Geometry: final body of the model. Coordinates: model frame, mm. A direction names the side the tool comes from. Coordinates: 2 decimals unless noted, no trailing zeros. Order: outer loops, then holes, each group sorted by start corner. A loop starts at its lowest first (then second) coordinate and runs counter-clockwise, first axis right, second up. Notation, with made-up numbers: (87.5, -4.75) - (141.5, -4.75) arc R20 cw to (141.5, 24.25) - close; hole circle Ø2 at (40.5, -12.75). An arc over 180 degrees is marked (long way). Use a Markdown table: item, result. Add a question column.
```python
from build123d import *

# Parameters (mm, degrees)
CROQUIS1_R              = 10
SALIENTE_EXTRUIR2_DEPTH = 50
CROQUIS4_R              = 30
SALIENTE_EXTRUIR3_DEPTH = 3
SALIENTE_EXTRUIR4_START = 25
CROQUIS5_R              = 30
SALIENTE_EXTRUIR4_DEPTH = 3
REDONDEO2_R             = 10
CORTAR_EXTRUIR1_START   = 50
CORTAR_EXTRUIR1_DEPTH   = 20
CORTAR_EXTRUIR2_START   = 50
CROQUIS7_W              = 3.5
CROQUIS7_H              = 7.2
CORTAR_EXTRUIR2_DEPTH   = 10
CORTAR_EXTRUIR3_START   = 1.785357468
CORTAR_EXTRUIR3_DEPTH   = 8.214642632
CORTAR_EXTRUIR4_START   = 25
CROQUIS9_R              = 2
CORTAR_EXTRUIR4_DEPTH   = 3
REDONDEO3_R             = 3


# Read off the part's stored shape, not the designer's step: Cortar-Extruir3
with BuildPart() as part:
    # Croquis1 → Saliente-Extruir2 (new body)
    with BuildSketch(Plane.XY):
        Circle(CROQUIS1_R)
    extrude(amount=SALIENTE_EXTRUIR2_DEPTH)

    # Croquis4 → Saliente-Extruir3 (add)
    with BuildSketch(Plane.XY):
        Circle(CROQUIS4_R)
    extrude(amount=SALIENTE_EXTRUIR3_DEPTH)

    # Croquis5 → Saliente-Extruir4 (add)
    with BuildSketch(Plane.XY.offset(SALIENTE_EXTRUIR4_START)):
        Circle(CROQUIS5_R)
    extrude(amount=SALIENTE_EXTRUIR4_DEPTH)

    # Redondeo2
    redondeo2_edges = [part.edges().sort_by_distance(p)[0] for p in [
        (-10, 0, 25),
        (-10, 0, 3),
    ]]
    fillet(redondeo2_edges, radius=REDONDEO2_R)

    # Croquis6 → Cortar-Extruir1 (cut)
    with BuildSketch(Plane.XY.offset(CORTAR_EXTRUIR1_START)):
        with BuildLine():
            Line((2, 1.5), (2, -1.5))
            ThreePointArc((2, -1.5), (-2.5, 0), (2, 1.5))
        make_face()
    extrude(amount=-CORTAR_EXTRUIR1_DEPTH, mode=Mode.SUBTRACT)

    # Croquis7 → Cortar-Extruir2 (cut)
    with BuildSketch(Plane.XY.offset(CORTAR_EXTRUIR2_START)):
        with Locations((5.5, 0)):
            Rectangle(CROQUIS7_W, CROQUIS7_H)
    extrude(amount=-CORTAR_EXTRUIR2_DEPTH, mode=Mode.SUBTRACT)

    # Cortar-Extruir3 outline → Cortar-Extruir3 (cut)
    with BuildSketch(Plane(origin=(0, 0, 0), x_dir=(0, 0, -1), z_dir=(1, 0, 0)).offset(CORTAR_EXTRUIR3_START)):
        with BuildLine():
            add(Edge.make_bspline(
                [(-43.250000008, 0), (-43.250010298, 0.457042806), (-43.439269311, 0.91355666), (-44.08377392, 1.559232298), (-44.536167579, 1.749638189), (-45.461098225, 1.750360744), (-45.914256169, 1.560125471), (-46.558728463, 0.916635921), (-46.75, 0.463408547), (-46.75, -0.463408547), (-46.559497121, -0.915462774), (-45.915045576, -1.559741953), (-45.458501244, -1.749734355), (-44.543528816, -1.750265056), (-44.088756623, -1.563446648), (-43.437067231, -0.912124478), (-43.250180582, -0.457964068), (-43.250000045, -0.000460382), (-43.250000003, -0.000230191), (-43.250000008, 0)],
                knots=[0.500062925, 0.500062925, 0.500062925, 0.500062925, 0.625, 0.625, 0.750000001, 0.750000001, 0.875000002, 0.875000002, 1.000000004, 1.000000004, 1.125000006, 1.125000006, 1.250000009, 1.250000009, 1.375000013, 1.375000013, 1.500000015, 1.500000015, 1.50006294, 1.50006294, 1.50006294, 1.50006294], degree=3))
        make_face()
    extrude(amount=CORTAR_EXTRUIR3_DEPTH, mode=Mode.SUBTRACT)

    # Croquis9 → Cortar-Extruir4 (cut)
    with BuildSketch(Plane.XY.offset(CORTAR_EXTRUIR4_START)):
        with Locations((25, 0)):
            Circle(CROQUIS9_R)
    extrude(amount=CORTAR_EXTRUIR4_DEPTH, mode=Mode.SUBTRACT)

    # Redondeo3
    redondeo3_edges = [part.edges().sort_by_distance(p)[0] for p in [
        (-10, 0, 28),
    ]]
    fillet(redondeo3_edges, radius=REDONDEO3_R)


solid = part.part
```
1) Draft query along X for faces 4 (the face through (-2.17, -9.76, 13.99)), 5 (the face through (-2, -2, 50)), 6 (the face through (23, 0, 26)). Return one class per face: pulls with the +X half, pulls with the -X half, needs draft (parallel to the pull), parting line crosses it, or undercut.
2) Set-up query: faces 1 (the face through (-29.97, 1.32, 26.48)), 2 (the face through (5, 3.6, 45)), 3 (the face through (6, -20, 3)). Return all of +Z, -Z, +X, -X, +Y, -Y with unobstructed straight access to the full face (end or side cutting, diameter ignored); none if empty.
3) Section A-A (x = 0). Return loops of the section in (y, z).
4) Section B-B (y = 0). Give the number of separate pieces and of enclosed holes in the cut face, then the cut area to 3 significant figures.
5) Pin query (flat end, axial travel): pin 1 (4 mm diameter, centred on x = 5.5, z = 44.5, fed in from -Y); pin 2 (2 mm diameter, centred on y = -1.5, z = 44, fed in from -X); pin 3 (3 mm diameter, centred on x = 0, y = 0, fed in from +Z). Return the tip coordinate at first contact, or that it passes through.
6) Ray query, line 1 along Z through (x, y) = (-23, -11); line 2 along X through (y, z) = (0, 37); line 3 along X through (y, z) = (-0.5, 40.5). Return the intervals inside material, ascending.
7) Section C-C (x = 25). Return loops of the section in (y, z), then the cut area to 3 significant figures.
8) Section D-D (z = 22). Return loops of the section in (x, y), then the cut area to 3 significant figures.
Values follow:
| question | item | result |
|---|---|---|
| 1 | face 4 | parting line crosses it |
| 1 | face 5 | needs draft |
| 1 | face 6 | undercut |
| 2 | face 1 | +Z, -Z |
| 2 | face 2 | +Z |
| 2 | face 3 | none |
| 3 | outline | (-30, 0) - (30, 0) - (30, 3) - (20, 3) arc R10 cw to (10, 13) - (10, 15) arc R10 cw to (20, 25) - (30, 25) - (30, 28) - (13, 28) arc R3 cw to (10, 31) - (10, 50) - (2.5, 50) - (2.5, 30) - (-2.5, 30) - (-2.5, 50) - (-10, 50) - (-10, 31) arc R3 cw to (-13, 28) - (-30, 28) - (-30, 25) - (-20, 25) arc R10 cw to (-10, 15) - (-10, 13) arc R10 cw to (-20, 3) - (-30, 3) - close |
| 4 | separate pieces | 4 |
| 4 | enclosed holes | 0 |
| 4 | area | 1,180 mm² |
| 5 | pin 1 | stops at y = -9.37 |
| 5 | pin 2 | stops at x = -9.99 |
| 5 | pin 3 | stops at z = 30 |
| 6 | line 1 | z = 0 to 3, 25 to 28 |
| 6 | line 2 | x = -10 to -2.5, 2 to 10 |
| 6 | line 3 | x = -9.99 to -2.45, 2 to 3.75, 7.25 to 9.99 |
| 7 | outline | (-16.58, 0) - (16.58, 0) - (16.58, 3) - (-16.58, 3) - close; (-16.58, 25) - (-2, 25) - (-2, 28) - (-16.58, 28) - close; (2, 25) - (16.58, 25) - (16.58, 28) - (2, 28) - close |
| 7 | area | 187 mm² |
| 8 | outline | circle Ø25.72 at (0, 0) |
| 8 | area | 519 mm² |
